Model file for the job. Use its own axes, mm. A direction names the side the tool comes from. Give positions to 0.01 mm unless a question says otherwise; leave off trailing zeros. Loops run counter-clockwise (first coordinate to the right, second up) from the corner with the lowest first, then second, coordinate; pieces in that order, holes last. Notation, with made-up numbers: M 0,-22 L 57,-22 A20 ccw 57,10 Z; hole C 78.5,-28 d2. An arc over 180 degrees is marked long. Answer in a Markdown table with one row per item.
```python
from build123d import *

# Parameters (mm, degrees)
ESBO_O1_W                = 80
ESBO_O1_H                = 70
RESSALTO_EXTRUS_O1_DEPTH = 9.525
ESBO_O2_R                = 16
CORTE_EXTRUS_O1_DEPTH    = 10
ESBO_O4_R                = 2.5
CORTE_EXTRUS_O3_DEPTH    = 23
ESBO_O5_R                = 2.78
CORTE_EXTRUS_O4_DEPTH    = 9.525


with BuildPart() as part:
    # Esboço1 → Ressalto-extrusão1 (new body)
    with BuildSketch(Plane.XY):
        Rectangle(ESBO_O1_W, ESBO_O1_H)
    extrude(amount=RESSALTO_EXTRUS_O1_DEPTH)

    # Esboço2 → Corte-extrusão1 (cut)
    with BuildSketch(Plane.XY.offset(9.525)):
        with Locations((0, 5)):
            Circle(ESBO_O2_R)
    extrude(amount=-CORTE_EXTRUS_O1_DEPTH, mode=Mode.SUBTRACT)

    # Esboço4 → Corte-extrusão3 (cut)
    with BuildSketch(Plane(origin=(0, 35, 0), x_dir=(1, 0, 0), z_dir=(0, 1, 0))):
        with Locations(Location((20, -4.7625, 0), (0, 0, 180))):
            Circle(ESBO_O4_R)
        with Locations(Location((0, -4.7625, 0), (0, 0, 180))):
            Circle(ESBO_O4_R)
        with Locations(Location((-20, -4.7625, 0), (0, 0, 180))):
            Circle(ESBO_O4_R)
    extrude(amount=-CORTE_EXTRUS_O3_DEPTH, mode=Mode.SUBTRACT)

    # Esboço5 → Corte-extrusão4 (cut)
    with BuildSketch(Plane.XY.offset(9.525)):
        with Locations((-20, -30.24)):
            Circle(ESBO_O5_R)
        with Locations((20, -30.24)):
            Circle(ESBO_O5_R)
    extrude(amount=-CORTE_EXTRUS_O4_DEPTH, mode=Mode.SUBTRACT)


solid = part.part
```
Q1. Probe probe 1 along X at (y, z) = (-30.5, 4.75); probe 2 along X at (y, z) = (13.5, 6.25); probe 3 along Z at (x, y) = (20, 26) (1 decimal). List the from-to ranges inside material, lowest first.
Reported:
| item | result |
|---|---|
| probe 1 | -40 to -22.77, -17.23 to 17.23, 22.77 to 40 |
| probe 2 | -40 to -22.01, -17.99 to -13.56, 13.56 to 17.99, 22.01 to 40 |
| probe 3 | 0 to 2.3, 7.3 to 9.5 |
Q2. Mould opens along X. For faces 3 (the face through (-40, 0, 5)), 4 (the face through (-20, 12, 5)), 5 (the face through (-1, -15, 0)) say: released by +X, released by -X, zero draft, split by the parting line, or undercut.
Reported:
| item | result |
|---|---|
| face 3 | released by -X |
| face 4 | undercut |
| face 5 | zero draft |
Q3. Saw through at D-D (y = -30.24). Give the cut face in (x, z) (3 decimals), and give its area (3 significant figures).
Reported:
| item | result |
|---|---|
| outline | M -40,0 L -22.78,0 L -22.78,9.525 L -40,9.525 Z; M -17.22,0 L 17.22,0 L 17.22,9.525 L -17.22,9.525 Z; M 22.78,0 L 40,0 L 40,9.525 L 22.78,9.525 Z |
| area | 656 mm² |
Q4. Drop flat-ended pins along their axis: pin 1 (4.5 mm diameter, centred on x = -20, y = -30.24, fed in from -Z); pin 2 (3 mm diameter, centred on x = 20, z = 4.76, fed in from +Y); pin 3 (2 mm diameter, centred on x = -5, y = -19.5, fed in from -Z); pin 4 (4 mm diameter, centred on x = 0, z = 4.76, fed in from +Y). Give the stop position or say it passes through.
Reported:
| item | result |
|---|---|
| pin 1 | through |
| pin 2 | y = 12 |
| pin 3 | z = 0 |
| pin 4 | y = -10.87 |
Q5. Saw through at B-B (y = 5). Give the cut face in (x, z) (3 decimals), and give its area (3 significant figures).
Reported:
| item | result |
|---|---|
| outline | M -40,0 L -16,0 L -16,9.525 L -40,9.525 Z; M 16,0 L 40,0 L 40,9.525 L 16,9.525 Z |
| area | 457 mm² |
Q6. 3-axis set-ups, long thin cutter, end or side, ignore diameter. For faces 1 (the face through (-22.777, -30.118, 4.829)), 2 (the face through (0.54, 28, 2.32)): which of +Z, -Z, +X, -X, +Y, -Y reach the whole face in a straight line?
Reported:
| item | result |
|---|---|
| face 1 | +Z, -Z |
| face 2 | +Y |
Q7. Saw through at A-A (x = 0). Give the cut face in (y, z) (1 decimal), and give its area (3 significant figures).
Reported:
| item | result |
|---|---|
| outline | M -35,0 L -11,0 L -11,9.5 L -35,9.5 Z; M 21,0 L 35,0 L 35,2.3 L 21,2.3 Z; M 21,7.3 L 35,7.3 L 35,9.5 L 21,9.5 Z |
| area | 292 mm² |
Q8. Saw through at C-C (x = -20). Give the cut face in (y, z) (1 decimal).
Reported:
| item | result |
|---|---|
| outline | M -35,0 L -33,0 L -33,9.5 L -35,9.5 Z; M -27.5,0 L 35,0 L 35,2.3 L 12,2.3 L 12,7.3 L 35,7.3 L 35,9.5 L -27.5,9.5 Z |
